from build123d import *

# Parameters (mm, degrees)
F0_R          = 6
F0_R_2        = 2
F1_DEPTH      = 5
F2_R          = 6
F3_DEPTH      = 5
F4_R          = 17.5
F5_DEPTH      = 6
F5_DEPTH_BACK = 6
F7_END_RADIUS = 12.5
F6_R          = 6
F7_REACH      = 59.6347554857
F9_DEPTH      = 25
F10_R         = 6
F10_R_2       = 2
F11_DEPTH     = 7.5


with BuildPart() as f1:
    # F0 (on Top) → F1 (new body)
    with BuildSketch(Plane.XY):
        Circle(F0_R)
        Polygon((-4.0414518843, 0), (-2.0207259422, 3.5), (2.0207259422, 3.5), (4.0414518843, 0), (2.0207259422, -3.5), (-2.0207259422, -3.5), align=None, mode=Mode.SUBTRACT)
        Polygon((2.0207259422, 3.5), (-2.0207259422, 3.5), (-4.0414518843, 0), (-2.0207259422, -3.5), (2.0207259422, -3.5), (4.0414518843, 0), align=None)
        Circle(F0_R_2, mode=Mode.SUBTRACT)
    extrude(amount=F1_DEPTH)

    # F2 (on face) → F3 (join)
    with BuildSketch(Plane.XY.offset(5)):
        Circle(F2_R)
        Polygon((-2.5149954402, 3.1635630654), (1.482228261, 3.7598314744), (3.9972237013, 0.5962684089), (2.5149954402, -3.1635630654), (-1.482228261, -3.7598314744), (-3.9972237013, -0.5962684089), align=None, mode=Mode.SUBTRACT)
    extrude(amount=F3_DEPTH)

    # F4 (on Right) → F5 (join, two sides)
    with BuildSketch(Plane.YZ) as f5_sk:
        with Locations((0, 25.1631926373)):
            Circle(F4_R)
        with BuildLine():
            ThreePointArc((0, 12.6631926373), (-8.8388347648, 34.0020274021), (12.5, 25.1631926373))
            ThreePointArc((12.5, 25.1631926373), (8.8388347648, 16.3243578724), (0, 12.6631926373))
        make_face(mode=Mode.SUBTRACT)
    extrude(amount=-F5_DEPTH)
    extrude(f5_sk.sketch, amount=F5_DEPTH_BACK)

    f7_end = (Plane(origin=(3, 0, 25.1631926373), x_dir=(0, 0, -1), z_dir=(-1, 0, 0)) * Cylinder(F7_END_RADIUS, 232.2145957139, mode=Mode.PRIVATE)).faces().sort_by_distance((3, -12.5, 25.1631926373))[0]
    # F6 (on Top) → F7 (join, up to the whole of a round face its end follows)
    with BuildSketch(Plane.XY):
        Circle(F6_R)
    f7_long = extrude(amount=F7_REACH, mode=Mode.PRIVATE)
    add(split(f7_long, bisect_by=f7_end, keep=Keep.ALL, mode=Mode.PRIVATE).solids().sort_by_distance((0, 0, 0))[0])

    # F8 (on face) → F9 (cut)
    with BuildSketch(Plane(origin=(0, 0, 0), x_dir=(1, 0, 0), z_dir=(0, 0, -1))):
        Polygon((2.0207259422, 3.5), (-2.0207259422, 3.5), (-4.0414518843, 0), (-2.0207259422, -3.5), (2.0207259422, -3.5), (4.0414518843, 0), align=None)
    extrude(amount=-F9_DEPTH, mode=Mode.SUBTRACT)

    # F10 (on face) → F11 (join)
    with BuildSketch(Plane(origin=(0, 0, 0), x_dir=(1, 0, 0), z_dir=(0, 0, -1))):
        Circle(F10_R)
        Circle(F10_R_2, mode=Mode.SUBTRACT)
    extrude(amount=-F11_DEPTH)


solid = f1.part
Design review of the part built by this model. Coordinates are the model's own, in mm. A direction names the side the tool comes from. Give positions to 0.01 mm unless a question says otherwise; leave off trailing zeros. Order: outer loops, then holes, each group sorted by start corner. A loop starts at its lowest first (then second) coordinate and runs counter-clockwise, first axis right, second up. Notation, with made-up numbers: (9.25, -21) - (56.25, -21) arc R14 ccw to (56.25, -17) - close; hole circle Ø9 at (33, 76). An arc over 180 degrees is marked (long way). Use CSV: the item, a comma, the result in double quotes. Start each with the question number.
Q1. For line 1 (Z direction, x = -3.25, y = 0); line 2 (X direction, y = 0, z = 2.5), list the stretches that pass through material, from the lowest coordinate up.
Q2. Machinability: for faces 1 (the face through (6, 11, 18)), 2 (the face through (0, 3.5, 10)), 3 (the face through (5.54, -2.3, 4.3)), which of the approach directions +Z, -Z, +X, -X, +Y, -Y give a long, thin tool a straight path to every point of the face, cutting with its end or side? Answer none if there is none.
Q3. Draft analysis for pull direction Z (two halves, no side actions). For faces 4 (the face through (3, 1.8, 10.3)), 5 (the face through (0, 2, 4)), 6 (the face through (3, 0, 0)), state which applies: pulls with the +Z half, pulls with the -Z half, needs draft (parallel to the pull), parting line crosses it, or undercut.
Q4. Take a section at A-A (y = -10). State the section outline as (x, z) points.
Q5. Take a section at C-C (y = -1). State the section outline as (x, z) points.
Q6. For P1, Ø1, axis at x = 1, z = 24, coming from the -Y side; P2, Ø3, axis at x = 2.5, z = 14, coming from the -Y side; P3, Ø3, axis at x = -1.5, y = 13.5, coming from the +Z side; P4, Ø3.5, axis at x = -0.5, y = 1, coming from the +Z side, all flat-tipped, find the tip position at first contact; note any pin that passes through.
Q7. Take a section at B-B (z = 23.5). State the section outline as (x, y) points.
Q8. Take a section at D-D (z = 7). State the section outline as (x, y) points, and give its area (3 significant figures).
Calculated:
1,line 1,"z = 0 to 7.5, 37.66 to 42.66"
1,line 2,"x = -6 to -2, 2 to 6"
2,face 1,"+Z, -Z, +X, +Y, -Y"
2,face 2,"none"
2,face 3,"-Z"
3,face 4,"undercut"
3,face 5,"needs draft"
3,face 6,"pulls with the -Z half"
4,outline,"(-6, 10.8) - (6, 10.8) - (6, 17.66) - (-6, 17.66) - close; (-6, 32.66) - (6, 32.66) - (6, 39.52) - (-6, 39.52) - close"
5,outline,"(-6, 7.69) - (-5.92, 7.69) - (-5.92, 0) - (-1.73, 0) - (-1.73, 7.5) - (-3.46, 7.5) - (-3.46, 12.7) - (-6, 12.7) - close; (-6, 37.62) - (6, 37.62) - (6, 42.63) - (-6, 42.63) - close; (1.73, 0) - (5.92, 0) - (5.92, 7.69) - (6, 7.69) - (6, 12.7) - (3.46, 12.7) - (3.46, 7.5) - (1.73, 7.5) - close"
6,P1,"stops at y = -17.49"
6,P2,"stops at y = -14.59"
6,P3,"stops at z = 37.9"
6,P4,"stops at z = 42.66"
7,outline,"(-6, -17.42) - (6, -17.42) - (6, -12.39) - (-6, -12.39) - close; (-6, 12.39) - (6, 12.39) - (6, 17.42) - (-6, 17.42) - close"
8,outline,"circle Ø12 at (0, 0); hole circle Ø4 at (0, 0)"
8,area,"101 mm²"
